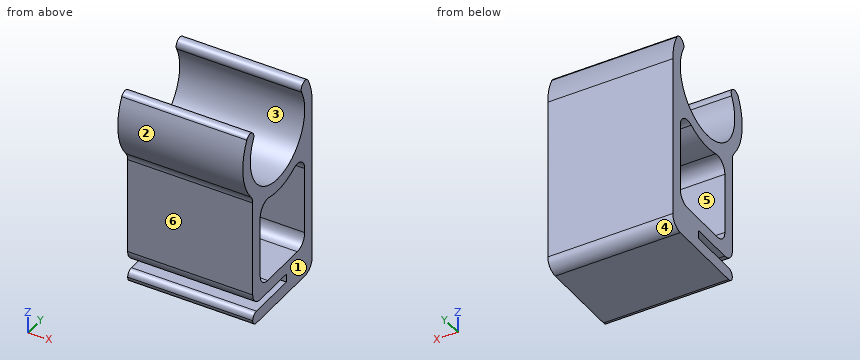
from build123d import *

# Parameters (mm, degrees)
F1_DEPTH = 15
F3_DEPTH = 30
F4_R     = 1.49999
F6_DEPTH = 30.001
F7_R     = 3


# Not quite as in the source:
# - a fillet or chamfer is up to 0.001 mm smaller than in the source, because OpenCascade refuses the exact size


with BuildPart() as f1:
    # F0 (on Right) → F1 (new body, symmetric)
    with BuildSketch(Plane.YZ):
        with BuildLine():
            ThreePointArc((12.3245305001, 6.4665811641), (10.2993352496, 7.0979164137), (9.668, 5.0727211632))
            ThreePointArc((9.668, 5.0727211632), (0, -10.918), (-9.668, 5.0727211632))
            ThreePointArc((-9.668, 5.0727211632), (-10.2993352496, 7.0979164137), (-12.3245305001, 6.4665811641))
            ThreePointArc((-12.3245305001, 6.4665811641), (0, -13.918), (12.3245305001, 6.4665811641))
        make_face()
    extrude(amount=F1_DEPTH, both=True)

    # F2 (on face) → F3 (join, through all)
    with BuildSketch(Plane.YZ.offset(15)):
        with BuildLine():
            ThreePointArc((13.918, 0), (5.2588084202, -12.886258495), (-9.944, -9.7379457793))
            Line((-9.944, -9.7379457793), (-9.944, -37.168))
            Line((-9.944, -37.168), (3.556, -37.168))
            Line((3.556, -37.168), (3.556, -39.168))
            Line((3.556, -39.168), (-9.944, -39.168))
            Line((-9.944, -39.168), (-9.944, -42.168))
            Line((-9.944, -42.168), (13.918, -42.168))
            Line((13.918, -42.168), (13.918, 0))
        make_face()
    extrude(amount=-F3_DEPTH)

    # F4 (radius 1.5 in the source; OpenCascade refuses exactly that, so slightly less here)
    f4_edges = [f1.edges().sort_by_distance(p)[0] for p in [
        (0, -9.944, -39.168),
        (0, -9.944, -42.168),
    ]]
    fillet(f4_edges, radius=F4_R)

    # F5 (on face) → F6 (cut, through all)
    with BuildSketch(Plane.YZ.offset(15)):
        with BuildLine():
            ThreePointArc((10.918, -8.6318016659), (2.6248268424, -13.6682481704), (-6.944, -12.0619893882))
            Line((-6.944, -12.0619893882), (-6.944, -34.168))
            Line((-6.944, -34.168), (10.918, -34.168))
            Line((10.918, -34.168), (10.918, -8.6318016659))
        make_face()
    extrude(amount=-F6_DEPTH, mode=Mode.SUBTRACT)

    # F7
    f7_edges = [f1.edges().sort_by_distance(p)[0] for p in [
        (0, -9.944, -9.737946),
        (0, -9.944, -37.168),
        (0, 13.918, -42.168),
        (0, -6.944, -12.061989),
        (0, 10.918, -8.631802),
        (0, 10.918, -34.168),
        (0, -6.944, -34.168),
    ]]
    fillet(f7_edges, radius=F7_R)


solid = f1.part
For this review, take the finished solid that the model builds, in its own axes (mm). Face numbers are marked on the shaded views. A direction names the side the tool comes from. Coordinates: 2 decimals unless noted, no trailing zeros. Loops run counter-clockwise (first coordinate to the right, second up) from the corner with the lowest first, then second, coordinate; pieces in that order, holes last. Notation, with made-up numbers: (54, 48) -> (88, 48) arc R24 cw to (88, 63) -> close; hole circle Ø8 at (-33.5, -20). An arc over 180 degrees is marked (long way). Write each question's results on one line, items separated by ' | '.
Q1. To check wall thickness, follow line 1 along Z through (x, y) = (7.75, -0.5); line 2 along Y through (x, z) = (-8.5, 0); line 3 along Z through (x, y) = (-8.25, -4.5). State the ranges of each line that lie inside material, in increasing order. Write a range as [from, to].
Taken from the geometry:
line 1: [-42.17, -39.17], [-37.17, -34.17], [-13.91, -10.91] | line 2: [-13.92, -10.92], [10.92, 13.92] | line 3: [-42.17, -39.17], [-37.17, -34.12], [-13.5, -9.95]
Q2. Add section A-A, the plane z = -19. State the section outline as (x, y) points, then the cut area to 3 significant figures.
Taken from the geometry:
outline: (-15, -9.94) -> (15, -9.94) -> (15, -6.94) -> (-15, -6.94) -> close; (-15, 10.92) -> (15, 10.92) -> (15, 13.92) -> (-15, 13.92) -> close | area: 180 mm²
Q3. Mouldability with a two-part tool opening along Y and no side actions: class the marked faces 1, 2 and 3 as +Y half, -Y half, draft (parallel to the pull), parting line (faces both ways), or undercut.
Taken from the geometry:
face 1: draft | face 2: -Y half | face 3: undercut
Q4. Add section C-C, the plane y = 4.75. State the section outline as (x, z) points.
Taken from the geometry:
outline: (-15, -42.17) -> (15, -42.17) -> (15, -34.17) -> (-15, -34.17) -> close; (-15, -13.08) -> (15, -13.08) -> (15, -9.83) -> (-15, -9.83) -> close
Q5. Machinability: for the marked faces 4, 5 and 6, which of the approach directions +Z, -Z, +X, -X, +Y, -Y give a long, thin tool a straight path to every point of the face, cutting with its end or side? Answer none if there is none.
Taken from the geometry:
face 4: -Z, +X, -X, +Y | face 5: +X, -X | face 6: -Z, +X, -X, -Y
Q6. Add section B-B, the plane y = 0. State the section outline as (x, z) points.
Taken from the geometry:
outline: (-15, -42.17) -> (15, -42.17) -> (15, -39.17) -> (-15, -39.17) -> close; (-15, -37.17) -> (15, -37.17) -> (15, -34.17) -> (-15, -34.17) -> close; (-15, -13.92) -> (15, -13.92) -> (15, -10.92) -> (-15, -10.92) -> close
Q7. For pin 1 Ø5 at (x, z) = (-1, -20) entering from -Y; pin 2 Ø9.5 at (x, y) = (-6, -1.5) entering from +Z; pin 3 Ø1 at (x, y) = (-10, -4.5) entering from +Z, all flat-tipped, find the tip position at first contact; note any pin that passes through.
Taken from the geometry:
pin 1: y = -9.94 | pin 2: z = -8.95 | pin 3: z = -9.71
